Study the drawing (mm; zero at the part's minimum x, y, z) and answer. A direction names the side the tool comes from. Give positions to 0.01 mm unless a question says otherwise; leave off trailing zeros. Order: outer loops, then holes, each group sorted by start corner. A loop starts at its lowest first (then second) coordinate and runs counter-clockwise, first axis right, second up.
Item 1: A cutting plane is placed at B-B (z = 1.25). Write down the section's boundary in (x, y).
Item 2: A cutting plane is placed at A-A (x = 13.5). Write down the section's boundary in (y, z).
Item 3: Find the intervals of material crossed by line 1 along Z through (x, y) = (13.5, 1.35); line 2 along Z through (x, y) = (2.75, 6.25); line 3 along Y through (x, z) = (15, 9.5), in increasing order.
Item 4: Given pin 1 Ø4 at (x, z) = (7.5, 8) entering from +Y; pin 2 Ø1.5 at (y, z) = (3, 7) entering from +X; pin 3 Ø2.5 at (y, z) = (3.5, 6) entering from -X, each flat-ended and moving along its own axis, determine where each tip first touches the part or whether it passes through.
Item 5: A cutting plane is placed at C-C (y = 9). Write down the section's boundary in (x, z).
Item 6: Which of the six approach directions +Z, -Z, +X, -X, +Y, -Y give full straight-line access (tool end or side, diameter ignored) to the marked faces 1, 2 and 3?
Item 7: The mould has two halves that part along Z. Classify the marked faces 4, 5 and 6: +Z half, -Z half, draft (parallel to the pull), parting line (faces both ways), or undercut.
Item 8: A cutting plane is placed at D-D (y = 2). Write down the section's boundary in (x, z).
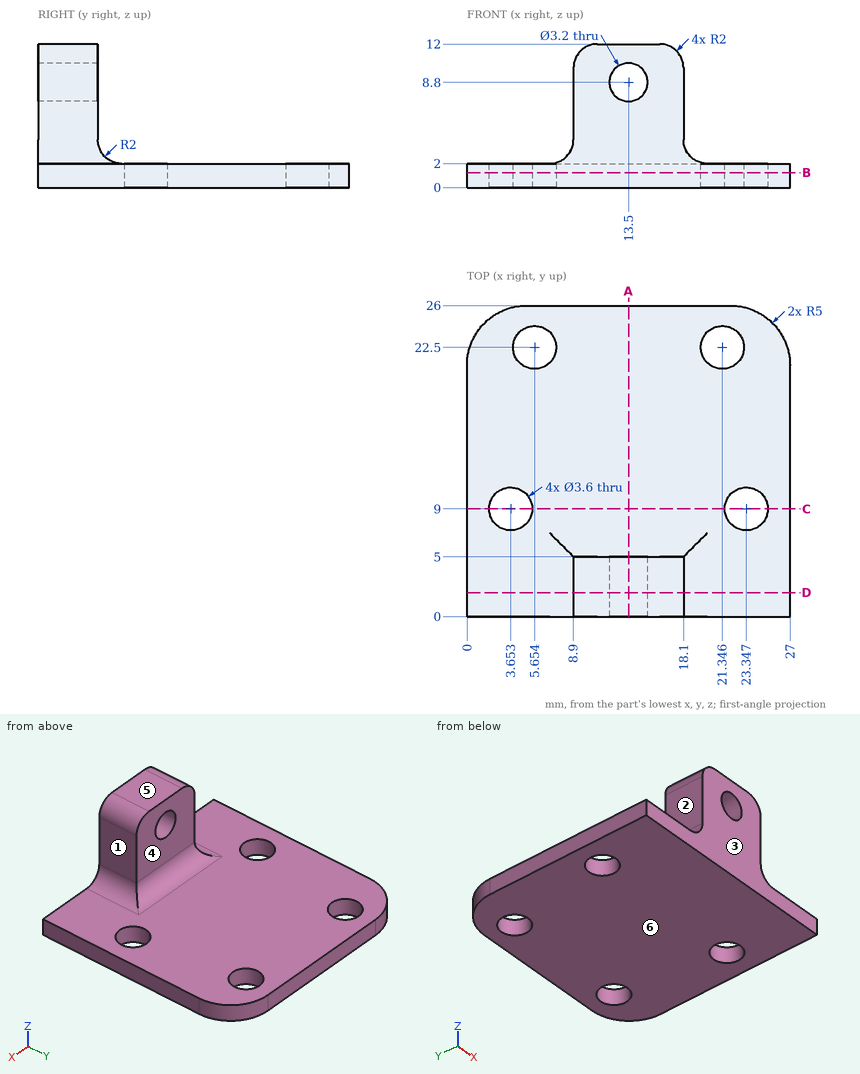
Response values:
1. outline: (0, 0) - (27, 0) - (27, 21) arc R5 ccw to (22, 26) - (5, 26) arc R5 ccw to (0, 21) - close; hole circle Ø3.6 at (3.65, 9); hole circle Ø3.6 at (5.65, 22.5); hole circle Ø3.6 at (21.35, 22.5); hole circle Ø3.6 at (23.35, 9)
2. outline: (0, 0) - (26, 0) - (26, 2) - (7, 2) arc R2 cw to (5, 4) - (5, 7.2) - (0, 7.2) - close; (0, 10.4) - (5, 10.4) - (5, 12) - (0, 12) - close
3. line 1: z = 0 to 7.2, 10.4 to 12
3. line 2: z = 0 to 2
3. line 3: y = 0 to 5
4. pin 1: stops at y = 5
4. pin 2: stops at x = 18.1
4. pin 3: stops at x = 8.9
5. outline: (0, 0) - (1.85, 0) - (1.85, 2) - (0, 2) - close; (5.45, 0) - (21.55, 0) - (21.55, 2) - (5.45, 2) - close; (25.15, 0) - (27, 0) - (27, 2) - (25.15, 2) - close
6. face 1: +Z, +X, +Y, -Y
6. face 2: +Z, -X, +Y, -Y
6. face 3: +Z, -Z, +X, -X, -Y
7. face 4: draft
7. face 5: +Z half
7. face 6: -Z half
8. outline: (0, 0) - (27, 0) - (27, 2) - (20.1, 2) arc R2 cw to (18.1, 4) - (18.1, 10) arc R2 ccw to (16.1, 12) - (10.9, 12) arc R2 ccw to (8.9, 10) - (8.9, 4) arc R2 cw to (6.9, 2) - (0, 2) - close; hole circle Ø3.2 at (13.5, 8.8)
